from build123d import *

# Parameters (mm, degrees)
BOSS_EXTRUDE2_DEPTH             = 118.925
BOSS_EXTRUDE1_REACH             = 140.65
SKETCH2_W                       = 18.25
SKETCH2_H                       = 43.65
BOSS_EXTRUDE1_DIRECTION_2_DEPTH = 20
CUT_EXTRUDE2_DEPTH              = 90
FILLET1_R                       = 10
FILLET2_R                       = 5
FILLET3_R                       = 1


with BuildPart() as part:
    # Sketch1 → Boss-Extrude2 (new, symmetric)
    with BuildSketch(Plane(origin=(0, 0, 0), x_dir=(0, 0, -1), z_dir=(1, 0, 0))):
        Polygon((0, 0), (-29.329393675, 50.8), (-36.329393675, 50.8), (-6.252899132, -12), (50, -7), (50, 0), align=None)
    extrude(amount=BOSS_EXTRUDE2_DEPTH, both=True)

    # Boss-Extrude1: up to this plane
    boss_extrude1_end = Plane(origin=(118.925, 0, 0), z_dir=(0, -0.5000000000000043, 0.8660254037844363))
    # Sketch2 → Boss-Extrude1 (add, up to the surface)
    with BuildSketch(Plane.XY, mode=Mode.PRIVATE) as boss_extrude1_sk1:
        with Locations((106.225, 25.4)):
            Rectangle(SKETCH2_W, SKETCH2_H)
    boss_extrude1_tool1 = split(extrude(boss_extrude1_sk1.sketch, amount=BOSS_EXTRUDE1_REACH, mode=Mode.PRIVATE), bisect_by=boss_extrude1_end, keep=Keep.BOTH, mode=Mode.PRIVATE)
    add(boss_extrude1_tool1.solids().sort_by_distance((106.225, 25.4, 0))[0])
    # Sketch2 → Boss-Extrude1 (add, up to the surface)
    with BuildSketch(Plane.XY, mode=Mode.PRIVATE) as boss_extrude1_sk2:
        with Locations((-106.225, 25.4)):
            Rectangle(SKETCH2_W, SKETCH2_H)
    boss_extrude1_tool2 = split(extrude(boss_extrude1_sk2.sketch, amount=BOSS_EXTRUDE1_REACH, mode=Mode.PRIVATE), bisect_by=boss_extrude1_end, keep=Keep.BOTH, mode=Mode.PRIVATE)
    add(boss_extrude1_tool2.solids().sort_by_distance((-106.225, 25.4, 0))[0])

    # Sketch2 → Boss-Extrude1 direction 2 (add)
    with BuildSketch(Plane.XY):
        with Locations((106.225, 25.4)):
            Rectangle(SKETCH2_W, SKETCH2_H)
        with Locations((-106.225, 25.4)):
            Rectangle(SKETCH2_W, SKETCH2_H)
    extrude(amount=-BOSS_EXTRUDE1_DIRECTION_2_DEPTH)

    # Sketch4 → Cut-Extrude2 (cut, symmetric)
    with BuildSketch(Plane(origin=(0, 0, 0), x_dir=(0, 0, -1), z_dir=(1, 0, 0))):
        Polygon((-26.729651832, 30.755649855), (-20, 34.641016151), (-14, 24.248711306), (-14, 4.176018579), align=None)
    extrude(amount=CUT_EXTRUDE2_DEPTH, both=True, mode=Mode.SUBTRACT)

    # Fillet1
    fillet1_edges = [part.edges().sort_by_distance(p)[0] for p in [
        (0, -12, 6.252899132),
    ]]
    fillet(fillet1_edges, radius=FILLET1_R)

    # Fillet2
    fillet2_edges = [part.edges().sort_by_distance(p)[0] for p in [
        (0, -7, -50),
    ]]
    fillet(fillet2_edges, radius=FILLET2_R)

    # Fillet3
    fillet3_edges = [part.edges().sort_by_distance(p)[0] for p in [
        (0, 50.8, 36.329393675),
    ]]
    fillet(fillet3_edges, radius=FILLET3_R)


solid = part.part
The model under review builds one solid part; all positions refer to its coordinate system, in mm. A direction names the side the tool comes from. Give positions to 0.01 mm unless a question says otherwise; leave off trailing zeros. Loops run counter-clockwise (first coordinate to the right, second up) from the corner with the lowest first, then second, coordinate; pieces in that order, holes last. Notation, with made-up numbers: (64, 25.5) -> (69, 25.5) arc R29 cw to (69, 57.5) -> close; hole circle Ø3 at (19.25, 60.25). An arc over 180 degrees is marked (long way). Answer as a JSON object with one key per item and string values. Group by question number.
Q1. Draft analysis for pull direction X (two halves, no side actions). For faces 1 (the flat face through (115.35, 30, -1)), 2 (the flat face through (1, 14, 14)), 3 (the cylindrical face through (1.665, -10.072, 5.253)), 4 (the flat face through (-97.1, 30, -2)), state which applies: pulls with the +X half, pulls with the -X half, needs draft (parallel to the pull), parting line crosses it, or undercut.
Q2. Take a section at D-D (y = 45). Write out the cut boundary in (x, z) (3 decimals).
Q3. Wall thickness on line 1 along X through (y, z) = (35, -10.5); line 2 along X through (y, z) = (29, 17) (3 decimals); line 3 along Y through (x, z) = (-8, -45.5): over which ranges is each line inside the solid? List them lowest first.
Q4. Take a section at A-A (x = -58.5). Write out the cut boundary in (y, z), plus the area to 3 significant figures.
Q5. Take a section at C-C (z = -13). Write out the cut boundary in (x, y) (3 decimals), plus the area to 3 significant figures.
Q6. Insertion check: pin 1 (2 mm diameter, centred on x = 5, z = -20.5, fed in from +Y); pin 2 (20 mm diameter, centred on x = 105, y = 18.5, fed in from -Z); pin 3 (1.5 mm diameter, centred on x = 26.5, y = 37, fed in from +Z); pin 4 (6 mm diameter, centred on y = 18, z = 10, fed in from +X) (3 decimals). Each pin has a flat end and moves straight along its axis. Give the tip position at first contact, or say it passes through.
Q7. Tool access review of faces 5 (the flat face through (-106, 26, -20)), 6 (the flat face through (97.1, 30, -1)), 7 (the flat face through (-106, 3.575, -9)), 8 (the flat face through (-115.35, 30, -2)), 9 (the flat face through (1.26, 32.67, 23.41)): name each direction out of +Z, -Z, +X, -X, +Y, -Y from which nothing blocks a thin tool from reaching the whole face with its end or side.
Q8. Take a section at B-B (z = 16.5). Write out the cut boundary in (x, y) (3 decimals), plus the area to 3 significant figures.
Answer below:
{
 "1": {"face 1": "pulls with the +X half", "face 2": "undercut", "face 3": "needs draft", "face 4": "undercut"},
 "2": {"outline": "(-118.925, 25.981) -> (-115.35, 25.981) -> (-115.35, -20) -> (-97.1, -20) -> (-97.1, 25.981) -> (97.1, 25.981) -> (97.1, -20) -> (115.35, -20) -> (115.35, 25.981) -> (118.925, 25.981) -> (118.925, 33.552) -> (-118.925, 33.552) -> close"},
 "3": {"line 1": "x = -115.35 to -97.1, 97.1 to 115.35", "line 2": "x = -118.925 to -90, 90 to 118.925", "line 3": "y = -7.4 to 0"},
 "4": {"outline": "(-11.39, -0.66) -> (-7.41, -45.44) arc R5 ccw to (-2.42, -50) -> (0, -50) -> (0, 0) -> (24.25, 14) -> (4.18, 14) -> (-5.74, 9.25) arc R10 ccw to start; (30.76, 26.73) -> (34.64, 20) -> (50.8, 29.33) -> (50.8, 34.74) arc R1 ccw to (49.37, 35.64) -> close", "area": "863 mm2"},
 "5": {"outline": "(-118.925, -10.289) -> (118.925, -10.289) -> (118.925, 0) -> (-118.925, 0) -> close; (-115.35, 3.575) -> (-97.1, 3.575) -> (-97.1, 47.225) -> (-115.35, 47.225) -> close; (97.1, 3.575) -> (115.35, 3.575) -> (115.35, 47.225) -> (97.1, 47.225) -> close", "area": "4,040 mm2"},
 "6": {"pin 1": "stops at y = 0", "pin 2": "stops at z = -20", "pin 3": "stops at z = 30.08", "pin 4": "stops at x = 118.925"},
 "7": {"face 5": "-Z, +X, -X, +Y", "face 6": "-Z, +Y", "face 7": "-Z, +X, -X", "face 8": "-Z, -X, +Y", "face 9": "-Z, -Y"},
 "8": {"outline": "(-118.925, 9.396) -> (-90, 9.396) -> (-90, 28.579) -> (-97.1, 28.579) -> (-97.1, 47.225) -> (-115.35, 47.225) -> (-115.35, 28.579) -> (-118.925, 28.579) -> close; (90, 9.396) -> (118.925, 9.396) -> (118.925, 28.579) -> (115.35, 28.579) -> (115.35, 47.225) -> (97.1, 47.225) -> (97.1, 28.579) -> (90, 28.579) -> close", "area": "1,790 mm2"}
}
